Read the model definition and answer for the solid it produces. Units are mm, in the model's axes. A direction names the side the tool comes from. Coordinates: 2 decimals unless noted, no trailing zeros. Loops run counter-clockwise (first coordinate to the right, second up) from the corner with the lowest first, then second, coordinate; pieces in that order, holes last.
Q1. Which of the six approach directions +Z, -Z, +X, -X, +Y, -Y give full straight-line access (tool end or side, diameter ignored) to faces 5 (the face through (6, -2.5, 10.9)), 6 (the face through (-4.43, 1.2, 10.95))?
Q2. Flat-ended cylindrical pins translate along their axes: P1, Ø3, axis at x = 0, y = 0, coming from the -Z side; P2, Ø1, axis at x = -6, y = 2.5, coming from the -Z side; P3, Ø3, axis at y = 0, z = 11, coming from the -X side; P4, Ø6, axis at x = 6.5, z = 4.5, coming from the -Y side. Find the tip coordinate at first contact, or state that the pin passes through.
Q3. Section A-A (z = 10.25) is taken. Give the vertices of the cut face in (x, y), then the cut area to 3 significant figures.
Q4. Straight lines are drawn through the part: line 1 (Y direction, x = 0, z = 2.8); line 2 (Y direction, x = -0.75, z = 1.5); line 3 (Z direction, x = -6.75, y = 8). For each, find the intervals that lie inside material, in ascending order.
Q5. Section B-B (x = 0) is taken. Give the vertices of the cut face in (y, z), then the cut area to 3 significant figures.
Q6. Section D-D (y = 10) is taken. Give the vertices of the cut face in (x, z).
Q7. Section C-C (y = 0) is taken. Give the vertices of the cut face in (x, z), then the cut area to 3 significant figures.
Q8. The mould has two halves that part along Z. Classify faces 1 (the face through (4.43, 1.2, 10.95)), 2 (the face through (0.854, -8.359, 3.042)), 3 (the face through (3, 0, 0)), 4 (the face through (6, 3, 6)): pulls with the +Z half, pulls with the -Z half, needs draft (parallel to the pull), parting line crosses it, or undercut.
from build123d import *

# Parameters (mm, degrees)
SKETCH2_R               = 13.5
BOSS_EXTRUDE1_DEPTH     = 6
SKETCH3_R               = 6.5
SKETCH3_R_2             = 2.5
BOSS_EXTRUDE2_DEPTH     = 10
SKETCH4_R               = 1.2
CUT_EXTRUDE1_DEPTH      = 25
CUT_EXTRUDE1_DEPTH_BACK = 25
SKETCH6_R               = 2.7
CUT_EXTRUDE3_DEPTH      = 50
CUT_EXTRUDE3_DEPTH_BACK = 20
SKETCH5_R               = 1.85
CUT_EXTRUDE4_DEPTH      = 10


with BuildPart() as part:
    # Sketch2 → Boss-Extrude1 (new body)
    with BuildSketch(Plane.XY):
        Circle(SKETCH2_R)
    extrude(amount=BOSS_EXTRUDE1_DEPTH)

    # Sketch3 → Boss-Extrude2 (add)
    with BuildSketch(Plane.XY.offset(6)):
        Circle(SKETCH3_R)
        Circle(SKETCH3_R_2, mode=Mode.SUBTRACT)
    extrude(amount=BOSS_EXTRUDE2_DEPTH)

    # Sketch4 → Cut-Extrude1 (cut, two sides)
    with BuildSketch(Plane(origin=(0, 0, 0), x_dir=(0, -1, 0), z_dir=(1, 0, 0))) as cut_extrude1_sk:
        with Locations((0, -11)):
            Circle(SKETCH4_R)
    extrude(amount=CUT_EXTRUDE1_DEPTH, mode=Mode.SUBTRACT)
    extrude(cut_extrude1_sk.sketch, amount=-CUT_EXTRUDE1_DEPTH_BACK, mode=Mode.SUBTRACT)

    # Sketch6 → Cut-Extrude3 (cut, two sides)
    with BuildSketch(Plane.XY.offset(6)) as cut_extrude3_sk:
        Circle(SKETCH6_R)
    extrude(amount=CUT_EXTRUDE3_DEPTH, mode=Mode.SUBTRACT)
    extrude(cut_extrude3_sk.sketch, amount=-CUT_EXTRUDE3_DEPTH_BACK, mode=Mode.SUBTRACT)

    # Sketch5 → Cut-Extrude4 (cut)
    with BuildSketch(Plane.XY.offset(6)):
        with Locations((0, 10)):
            Circle(SKETCH5_R)
    cut_extrude4 = extrude(amount=-CUT_EXTRUDE4_DEPTH, mode=Mode.SUBTRACT)

    # Mirror1: Cut-Extrude4 across plane
    add(cut_extrude4.mirror(Plane.ZX), mode=Mode.SUBTRACT)


solid = part.part
Numbers:
1. face 5: +Z
1. face 6: +X, -X
2. P1: passes through
2. P2: stops at z = 0
2. P3: stops at x = -6.5
2. P4: stops at y = -13.04
3. outline: (-6.43, -0.94) arc R6.5 ccw to (6.43, -0.94) - (2.53, -0.94) arc R2.7 cw to (-2.53, -0.94) - close; (-6.43, 0.94) - (-2.53, 0.94) arc R2.7 cw to (2.53, 0.94) - (6.43, 0.94) arc R6.5 ccw to start
3. area: 95.5 mm2
4. line 1: y = -13.5 to -11.85, -8.15 to -2.7, 2.7 to 8.15, 11.85 to 13.5
4. line 2: y = -13.48 to -11.69, -8.31 to -2.59, 2.59 to 8.31, 11.69 to 13.48
4. line 3: z = 0 to 6
5. outline: (-13.5, 0) - (-11.85, 0) - (-11.85, 6) - (-13.5, 6) - close; (-8.15, 0) - (-2.7, 0) - (-2.7, 16) - (-6.5, 16) - (-6.5, 6) - (-8.15, 6) - close; (2.7, 0) - (8.15, 0) - (8.15, 6) - (6.5, 6) - (6.5, 16) - (2.7, 16) - close; (11.85, 0) - (13.5, 0) - (13.5, 6) - (11.85, 6) - close
5. area: 161 mm2
6. outline: (-9.07, 0) - (-1.85, 0) - (-1.85, 6) - (-9.07, 6) - close; (1.85, 0) - (9.07, 0) - (9.07, 6) - (1.85, 6) - close
7. outline: (-13.5, 0) - (-2.7, 0) - (-2.7, 9.8) - (-6.5, 9.8) - (-6.5, 6) - (-13.5, 6) - close; (-6.5, 12.2) - (-2.7, 12.2) - (-2.7, 16) - (-6.5, 16) - close; (2.7, 0) - (13.5, 0) - (13.5, 6) - (6.5, 6) - (6.5, 9.8) - (2.7, 9.8) - close; (2.7, 12.2) - (6.5, 12.2) - (6.5, 16) - (2.7, 16) - close
7. area: 187 mm2
8. face 1: undercut
8. face 2: needs draft
8. face 3: pulls with the -Z half
8. face 4: pulls with the +Z half
